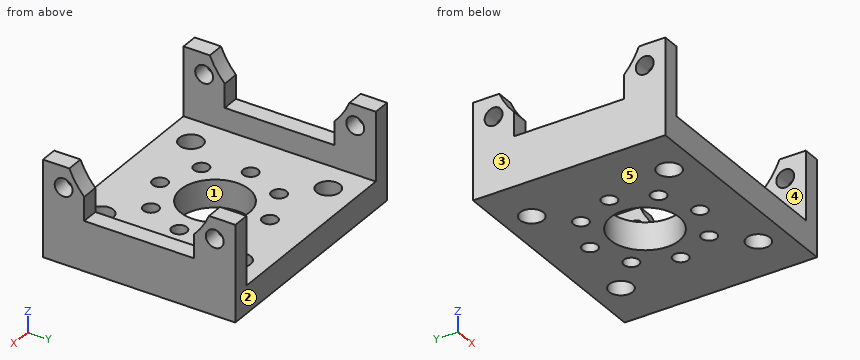
from build123d import *

# Parameters (mm, degrees)
SKETCH_W        = 34
SKETCH_H        = 28
PAD_DEPTH       = 4
SKETCH001_W     = 2.5
SKETCH001_H     = 28
PAD001_DEPTH    = 10
SKETCH002_R     = 1.3
POCKET_DEPTH    = 100
POCKET003_DEPTH = 100
SKETCH004_R     = 1.1
SKETCH004_R_2   = 5
POCKET007_DEPTH = 5
SKETCH008_R     = 1.7
POCKET009_DEPTH = 10


with BuildPart() as part:
    # Sketch → Pad (new body)
    with BuildSketch(Plane.XY):
        Rectangle(SKETCH_W, SKETCH_H)
    extrude(amount=PAD_DEPTH)

    # Sketch001 (on Face6 of Pad) → Pad001 (join)
    with BuildSketch(Plane.XY.offset(4)):
        with Locations((15.75, 0)):
            Rectangle(SKETCH001_W, SKETCH001_H)
        with Locations((-15.75, 0)):
            Rectangle(SKETCH001_W, SKETCH001_H)
    extrude(amount=PAD001_DEPTH)

    # Sketch002 (on Face13 of Pad001) → Pocket (cut)
    with BuildSketch(Plane.YZ.offset(17)):
        with Locations((-11, 11)):
            Circle(SKETCH002_R)
        with Locations((11, 11)):
            Circle(SKETCH002_R)
    extrude(amount=-POCKET_DEPTH, mode=Mode.SUBTRACT)

    # Sketch006 → Pocket003 (cut)
    with BuildSketch(Plane(origin=(-20, 0, 0), x_dir=(0, -1, 0), z_dir=(-1, 0, 0))):
        with BuildLine():
            ThreePointArc((8, 10.650166), (0, 29.2), (-8, 10.650166))
            Line((-8, 10.650166), (-8, 7.2))
            Line((-8, 7.2), (8, 7.2))
            Line((8, 7.2), (8, 10.650166))
        make_face()
    extrude(amount=-POCKET003_DEPTH, mode=Mode.SUBTRACT)

    # Sketch004 → Pocket007 (cut)
    with BuildSketch(Plane.XY.offset(4)):
        with Locations((0, 8)):
            Circle(SKETCH004_R)
        with Locations((8, 0)):
            Circle(SKETCH004_R)
        with Locations((0, -8)):
            Circle(SKETCH004_R)
        with Locations((-8, 0)):
            Circle(SKETCH004_R)
        Circle(SKETCH004_R_2)
        with Locations((5.656854, 5.656854)):
            Circle(SKETCH004_R)
        with Locations((-5.656854, 5.656854)):
            Circle(SKETCH004_R)
        with Locations((-5.656854, -5.656854)):
            Circle(SKETCH004_R)
        with Locations((5.656854, -5.656854)):
            Circle(SKETCH004_R)
    extrude(amount=-POCKET007_DEPTH, mode=Mode.SUBTRACT)

    # Sketch008 → Pocket009 (cut)
    with BuildSketch(Plane(origin=(0, 0, 0), x_dir=(1, 0, 0), z_dir=(0, 0, -1))):
        with Locations((10, 10)):
            Circle(SKETCH008_R)
        with Locations((-10, 10)):
            Circle(SKETCH008_R)
        with Locations((-10, -10)):
            Circle(SKETCH008_R)
        with Locations((10, -10)):
            Circle(SKETCH008_R)
    extrude(amount=-POCKET009_DEPTH, mode=Mode.SUBTRACT)


solid = part.part
The listing builds one solid part. Answer for the finished solid, in the listing's coordinates (mm). Face numbers are marked on the shaded views. A direction names the side the tool comes from. Round coordinates to 2 decimals unless told otherwise and drop trailing zeros. Write each loop counter-clockwise with the first axis right and the second up, starting at its lowest first coordinate (ties: lowest second). Pieces come first, ordered by that corner, then holes. Notation, with made-up numbers: (3, -3) - (39, -3) arc R23 ccw to (39, 23) - close; hole circle Ø10 at (89, 85). An arc over 180 degrees is marked (long way). Use a Markdown table: item, result. Add a question column.
1. The part is cut by section D-D (y = 11). Write down the section's boundary in (x, z).
2. Consider line 1 (Y direction, x = -10, z = 2.8); line 2 (X direction, y = 11.75, z = 6.75); line 3 (X direction, y = -6.5, z = 0.75). Determine where each line is inside the solid, lowest interval first.
3. Flat-ended cylindrical pins translate along their axes: P1, Ø1.8, axis at x = 5.66, y = -5.66, coming from the -Z side; P2, Ø3, axis at x = -12.5, y = -5.5, coming from the +Z side. Find the tip coordinate at first contact, or state that the pin passes through.
4. The part is cut by section A-A (z = 5.5). Write down the section's boundary in (x, y).
5. For a pull along X with two mould halves and no side action, classify the marked faces 1, 2 and 3 as +X half, -X half, draft (parallel to the pull), parting line (faces both ways), or undercut.
6. The part is cut by section C-C (x = 15.5). Write down the section's boundary in (y, z), and give its area (3 significant figures).
7. The part is cut by section B-B (x = -10). Write down the section's boundary in (y, z).
8. A tool of negligible diameter and unlimited length cuts with its end or side. For the marked faces 4 and 5, from which of +Z, -Z, +X, -X, +Y, -Y can it reach the whole face along a straight path? Write none if from no direction.
Reported:
| question | item | result |
|---|---|---|
| 1 | outline | (-17, 0) - (-11.37, 0) - (-11.37, 4) - (-14.5, 4) - (-14.5, 9.7) - (-17, 9.7) - close; (-17, 12.3) - (-14.5, 12.3) - (-14.5, 14) - (-17, 14) - close; (-8.63, 0) - (8.63, 0) - (8.63, 4) - (-8.63, 4) - close; (11.37, 0) - (17, 0) - (17, 9.7) - (14.5, 9.7) - (14.5, 4) - (11.37, 4) - close; (14.5, 12.3) - (17, 12.3) - (17, 14) - (14.5, 14) - close |
| 2 | line 1 | -14 to -11.7, -8.3 to 8.3, 11.7 to 14 |
| 2 | line 2 | -17 to -14.5, 14.5 to 17 |
| 2 | line 3 | -17 to -6.36, -4.95 to 4.95, 6.36 to 17 |
| 3 | P1 | through |
| 3 | P2 | z = 4 |
| 4 | outline | (-17, -14) - (-14.5, -14) - (-14.5, 14) - (-17, 14) - close; (14.5, -14) - (17, -14) - (17, 14) - (14.5, 14) - close |
| 5 | face 1 | undercut |
| 5 | face 2 | draft |
| 5 | face 3 | -X half |
| 6 | outline | (-14, 0) - (14, 0) - (14, 14) - (10.17, 14) arc R11 cw to (8, 10.65) - (8, 7.2) - (-8, 7.2) - (-8, 10.65) arc R11 cw to (-10.17, 14) - (-14, 14) - close; hole circle Ø2.6 at (-11, 11); hole circle Ø2.6 at (11, 11) |
| 6 | area | 264 mm^2 |
| 7 | outline | (-14, 0) - (-11.7, 0) - (-11.7, 4) - (-14, 4) - close; (-8.3, 0) - (8.3, 0) - (8.3, 4) - (-8.3, 4) - close; (11.7, 0) - (14, 0) - (14, 4) - (11.7, 4) - close |
| 8 | face 4 | +Z, +Y, -Y |
| 8 | face 5 | -Z, +X, -X, +Y, -Y |
